Geometry check sheet. Reference: the model listing, model coordinates, mm. A direction names the side the tool comes from. Round coordinates to 2 decimals unless told otherwise and drop trailing zeros. Loops run counter-clockwise (first coordinate to the right, second up) from the corner with the lowest first, then second, coordinate; pieces in that order, holes last. Notation, with made-up numbers: M 52.5,73.25 L 57.5,73.25 A19 ccw 57.5,84.25 Z; hole C 17.5,-2 d6. An arc over 180 degrees is marked long. Answer in a Markdown table with one row per item. Add a question column.
```python
from build123d import *

# Parameters (mm, degrees)
SKETCH1_R           = 11
BOSS_EXTRUDE1_DEPTH = 3.5
SKETCH2_R           = 4
CUT_EXTRUDE3_DEPTH  = 6
CIRPATTERN1_COUNT   = 8


with BuildPart() as part:
    # Sketch1 → Boss-Extrude1 (new body, symmetric)
    with BuildSketch(Plane.XY):
        Polygon((7.870057685, 19), (-7.870057685, 19), (-19, 7.870057685), (-19, -7.870057685), (-7.870057685, -19), (7.870057685, -19), (19, -7.870057685), (19, 7.870057685), align=None)
        Circle(SKETCH1_R, mode=Mode.SUBTRACT)
    extrude(amount=BOSS_EXTRUDE1_DEPTH, both=True)

    # Sketch2 → Cut-Extrude3 (cut)
    with BuildSketch(Plane(origin=(0, -19, 0), x_dir=(-1, 0, 0), z_dir=(0, -1, 0))):
        Circle(SKETCH2_R)
    cut_extrude3 = extrude(amount=-CUT_EXTRUDE3_DEPTH, mode=Mode.SUBTRACT)

    # CirPattern1: Cut-Extrude3 ×8 about axis
    cirpattern1_axis = Axis((0, 0, 0), (0, 0, 1))
    for i in range(1, CIRPATTERN1_COUNT):
        add(cut_extrude3.rotate(cirpattern1_axis, i * 360 / CIRPATTERN1_COUNT), mode=Mode.SUBTRACT)


solid = part.part
```
1) Cross-section at C-C, the plane x = 11.5. Count the separate pieces of the cut face and the enclosed holes in it, plus the area to 3 significant figures.
2) Draft check along X on faces 3 (the flat face through (9.53, 17.34, 0.05)), 4 (the cylindrical face through (14.172, -8.515, -0.06)), 5 (the flat face through (-6, 19, 0)). Enter one of: +X half, -X half, draft (parallel to the pull), parting line (faces both ways), or undercut.
3) Cross-section at A-A, the plane x = 0. Record the boundary of the cut face in (y, z), plus the area to 3 significant figures.
4) Go/stop test with flat-tipped pins: pin 1 (4 mm diameter, centred on y = 1, z = 0, fed in from -X); pin 2 (2 mm diameter, centred on x = 0, z = 0, fed in from +Y); pin 3 (4 mm diameter, centred on x = 15, z = 1, fed in from +Y). Record where each tip stops, or that it passes through.
5) Set-up check for faces 1 (the flat face through (-13, 0, 0)), 2 (the flat face through (-17.34, 9.53, 0.05)): record each of +Z, -Z, +X, -X, +Y, -Y from which the full face is reachable in a straight line by a thin tool's end or side.
6) Thickness scan on L1, parallel to Y at x = 0, z = 1.5; L2, parallel to X at y = 7, z = 2; L3, parallel to Y at x = -9.5, z = 1. Record the ranges inside material, lowest first. Write a range as [from, to].
Worked answers:
| question | item | result |
|---|---|---|
| 1 | separate pieces | 5 |
| 1 | enclosed holes | 0 |
| 1 | area | 101 mm2 |
| 2 | face 3 | +X half |
| 2 | face 4 | undercut |
| 2 | face 5 | draft |
| 3 | outline | M -13,-3.5 L -11,-3.5 L -11,3.5 L -13,3.5 Z; M 11,-3.5 L 13,-3.5 L 13,3.5 L 11,3.5 Z |
| 3 | area | 28.0 mm2 |
| 4 | pin 1 | stops at x = -13 |
| 4 | pin 2 | stops at y = 13 |
| 4 | pin 3 | stops at y = 11.54 |
| 5 | face 1 | -X |
| 5 | face 2 | +Z, -Z, -X, +Y |
| 6 | L1 | y = [-13, -11], [11, 13] |
| 6 | L2 | x = [-19, -11.9], [-11.38, -8.49], [8.49, 11.38], [11.9, 19] |
| 6 | L3 | y = [-17.37, -14.98], [-8.88, -5.55], [5.55, 8.88], [14.98, 17.37] |
